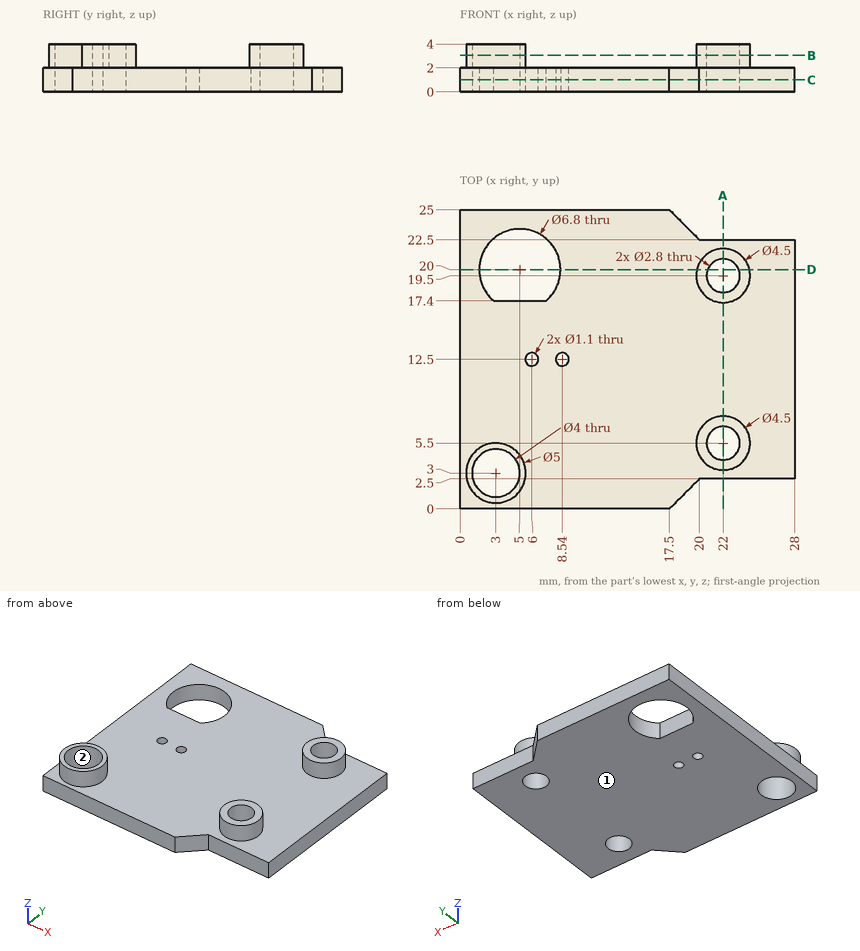
Answer from the drawing. Dimensions are ordinates in mm from the lowest x, y and z of the part. Give positions to 0.01 mm unless a question says otherwise; leave off trailing zeros. Loops run counter-clockwise (first coordinate to the right, second up) from the corner with the lowest first, then second, coordinate; pieces in that order, holes last.
Item 1: A cutting plane is placed at D-D (y = 20). Give the vertices of the cut face in (x, z).
Derived:
outline: (0, 0) - (1.6, 0) - (1.6, 2) - (0, 2) - close; (8.4, 0) - (20.69, 0) - (20.69, 4) - (19.81, 4) - (19.81, 2) - (8.4, 2) - close; (23.31, 0) - (28, 0) - (28, 2) - (24.19, 2) - (24.19, 4) - (23.31, 4) - close
Item 2: Determine the mould class of the marked faces 1 and 2 for opening direction Y: +Y half, -Y half, draft (parallel to the pull), parting line (faces both ways), or undercut.
Derived:
face 1: draft
face 2: undercut
Item 3: Find the intervals of material crossed by line 1 along Y through (x, z) = (22, 2.8); line 2 along X through (y, z) = (20, 1.2); line 3 along Y through (x, z) = (6, 1.25), in increasing order.
Derived:
line 1: y = 3.25 to 4.1, 6.9 to 7.75, 17.25 to 18.1, 20.9 to 21.75
line 2: x = 0 to 1.6, 8.4 to 20.69, 23.31 to 28
line 3: y = 0 to 11.95, 13.05 to 17.4, 23.25 to 25
Item 4: Each of these flat-tipped pins is pushed along its axis until it touches: pin 1 Ø12.5 at (x, y) = (13.5, 16) entering from +Z; pin 2 Ø1.6 at (x, z) = (25, 1.5) entering from +Y; pin 3 Ø1 at (y, z) = (5.5, 3) entering from -X. Where does it stop, or does it pass through?
Derived:
pin 1: stops at z = 2
pin 2: stops at y = 22.5
pin 3: stops at x = 1.5
Item 5: A cutting plane is placed at A-A (x = 22). Give the vertices of the cut face in (y, z).
Derived:
outline: (2.5, 0) - (4.1, 0) - (4.1, 4) - (3.25, 4) - (3.25, 2) - (2.5, 2) - close; (6.9, 0) - (18.1, 0) - (18.1, 4) - (17.25, 4) - (17.25, 2) - (7.75, 2) - (7.75, 4) - (6.9, 4) - close; (20.9, 0) - (22.5, 0) - (22.5, 2) - (21.75, 2) - (21.75, 4) - (20.9, 4) - close
Item 6: A cutting plane is placed at C-C (z = 1). Give the vertices of the cut face in (x, y).
Derived:
outline: (0, 0) - (17.5, 0) - (20, 2.5) - (28, 2.5) - (28, 22.5) - (20, 22.5) - (17.5, 25) - (0, 25) - close; hole circle Ø4 at (3, 3); hole (2.81, 17.4) - (7.19, 17.4) arc R3.4 ccw (long way) to start; hole circle Ø1.1 at (6, 12.5); hole circle Ø1.1 at (8.54, 12.5); hole circle Ø2.8 at (22, 5.5); hole circle Ø2.8 at (22, 19.5)
Item 7: A cutting plane is placed at B-B (z = 3.05). Give the vertices of the cut face in (x, y).
Derived:
outline: circle Ø5 at (3, 3); circle Ø4.5 at (22, 5.5); circle Ø4.5 at (22, 19.5); hole circle Ø4 at (3, 3); hole circle Ø2.8 at (22, 5.5); hole circle Ø2.8 at (22, 19.5)
